Can you work these out from the model? Positions are in its coordinate system, mm. A direction names the side the tool comes from. Round coordinates to 2 decimals unless told otherwise and drop trailing zeros. Order: outer loops, then holes, each group sorted by start corner. A loop starts at its lowest first (then second) coordinate and runs counter-clockwise, first axis right, second up. Notation, with made-up numbers: M -23,69 L -7,69 A17 ccw -7,94 Z; hole C -38.75,-34 d7. An arc over 180 degrees is marked long. Answer as a JSON object with one key per item and string values. Group by question number.
```python
from build123d import *

# Parameters (mm, degrees)
SKETCH2_R           = 7.5
BOSS_EXTRUDE1_DEPTH = 8
BOSS_EXTRUDE3_DEPTH = 8
SKETCH3_4_R         = 25
SKETCH3_4_R_2       = 15
BOSS_EXTRUDE4_DEPTH = 58
SKETCH17_W          = 8
SKETCH17_H          = 39.501765498
BOSS_EXTRUDE6_DEPTH = 78
CUT_EXTRUDE1_DEPTH  = 78


with BuildPart() as part:
    # Sketch2 → Boss-Extrude1 (new body)
    with BuildSketch(Plane(origin=(0, 0, 0), x_dir=(1, 0, 0), z_dir=(0, 1, 0))):
        with BuildLine():
            Line((-4.545115865, -26.622255639), (58.454884135, -26.622255639))
            ThreePointArc((58.454884135, -26.622255639), (69.061485853, -22.228857357), (73.454884135, -11.622255639))
            Line((73.454884135, -11.622255639), (73.454884135, 48.377744361))
            ThreePointArc((73.454884135, 48.377744361), (69.061485853, 58.984346079), (58.454884135, 63.377744361))
            Line((58.454884135, 63.377744361), (-4.545115865, 63.377744361))
            Line((-4.545115865, 63.377744361), (-4.545115865, -26.622255639))
        make_face()
        with Locations((58.454884135, -11.622255639)):
            Circle(SKETCH2_R, mode=Mode.SUBTRACT)
        with Locations((58.454884135, 48.377744361)):
            Circle(SKETCH2_R, mode=Mode.SUBTRACT)
    extrude(amount=BOSS_EXTRUDE1_DEPTH)

    # Sketch3 → Boss-Extrude3 (add)
    with BuildSketch(Plane.ZY.offset(4.545115865)):
        with BuildLine():
            Line((-18.377744361, 42), (-18.377744361, 8))
            Line((-18.377744361, 8), (26.622255639, 8))
            Line((26.622255639, 8), (6.622255639, 67))
            ThreePointArc((6.622255639, 67), (-0.700074831, 49.32233047), (-18.377744361, 42))
        make_face()
        with BuildLine():
            Line((-63.377744361, 8), (-18.377744361, 8))
            Line((-18.377744361, 8), (-18.377744361, 42))
            ThreePointArc((-18.377744361, 42), (-36.055413891, 49.32233047), (-43.377744361, 67))
            Line((-43.377744361, 67), (-63.377744361, 8))
        make_face()
    extrude(amount=-BOSS_EXTRUDE3_DEPTH)

    # Sketch3_4 → Boss-Extrude4 (add)
    with BuildSketch(Plane.ZY.offset(4.545115865)):
        with Locations((-18.377744361, 67)):
            Circle(SKETCH3_4_R)
        with Locations((-18.377744361, 67)):
            Circle(SKETCH3_4_R_2, mode=Mode.SUBTRACT)
    extrude(amount=-BOSS_EXTRUDE4_DEPTH)

    # Sketch17 → Boss-Extrude6 (add)
    with BuildSketch(Plane.ZY.offset(4.545115865)):
        with Locations((-18.377744361, 27.750882749)):
            Rectangle(SKETCH17_W, SKETCH17_H)
    extrude(amount=-BOSS_EXTRUDE6_DEPTH)

    # Sketch18 → Cut-Extrude1 (cut)
    with BuildSketch(Plane(origin=(0, 0, -22.377744361), x_dir=(-1, 0, 0), z_dir=(0, 0, -1))):
        Polygon((-73.454884135, 8), (-53.454884135, 42.322074641), (-53.454884135, 47.501765498), (-73.454884135, 47.501765498), align=None)
    extrude(amount=-CUT_EXTRUDE1_DEPTH, mode=Mode.SUBTRACT)


solid = part.part
```
1) Which directions (+Z, -Z, +X, -X, +Y, -Y) give clear straight access to the entire face, cutting with the end or side of a thin tool? Please do faces 4 (the face through (24.05, 91.98, -17.33)), 5 (the face through (3.455, 31, -39)), 6 (the face through (30, 25, -14.378)).
2) For pin 1 (6 mm diameter, centred on x = 9, y = 45, fed in from +Z); pin 2 (20.5 mm diameter, centred on y = 33.5, z = -40, fed in from +X); pin 3 (18 mm diameter, centred on y = 67, z = -18.38, fed in from -X); pin 4 (17 mm diameter, centred on x = 43.5, y = 20, fed in from -Z), each with a flat end and sliding along its axis, tell me the tip position at first contact or that it passes through.
3) If we section it at B-B on z = -11.5: Write out the boundary of the cut face in (x, y), plus the area to 3 significant figures.
4) We'd pull the mould along Y, two halves only. Please class faces 1 (the face through (-0.6, 37.91, -53.24)), 2 (the face through (34, 0, -19)), 3 (the face through (24.049, 52.357, -21.629)): +Y half, -Y half, draft (parallel to the pull), parting line (faces both ways), or undercut.
5) If we section it at C-C on y = 75: Write out the boundary of the cut face in (x, z), plus the area to 3 significant figures.
6) If we section it at A-A on x = 6.5: Write out the boundary of the cut face in (y, z).
7) I need wall thicknesses on line 1 along Y through (x, z) = (4, -24); line 2 along Y through (x, z) = (24.5, -28); line 3 along X through (y, z) = (33, -27.5). Which ranges of each line are inside material? Lowest first, please.
8) If we section it at D-D on x = 55: Write out the boundary of the cut face in (y, z), plus the area to 3 significant figures.
Findings:
{
 "1": {"face 4": "+X", "face 5": "-Z, +X", "face 6": "+Z, +X"},
 "2": {"pin 1": "stops at z = -2.13", "pin 2": "stops at x = 3.45", "pin 3": "passes through", "pin 4": "stops at z = -22.38"},
 "3": {"outline": "M -4.55,0 L 73.45,0 L 73.45,8 L 3.45,8 L 3.45,42.96 L 53.45,42.96 L 53.45,53.67 L -4.55,53.67 Z; M -4.55,80.33 L 53.45,80.33 L 53.45,91.04 L -4.55,91.04 Z", "area": "2,150 mm^2"},
 "4": {"face 1": "+Y half", "face 2": "-Y half", "face 3": "undercut"},
 "5": {"outline": "M -4.55,-42.06 L 53.45,-42.06 L 53.45,-31.07 L -4.55,-31.07 Z; M -4.55,-5.69 L 53.45,-5.69 L 53.45,5.31 L -4.55,5.31 Z", "area": "1,280 mm^2"},
 "6": {"outline": "M 0,-63.38 L 8,-63.38 L 8,-22.38 L 42.32,-22.38 A25 ccw long 42.32,-14.38 L 8,-14.38 L 8,26.62 L 0,26.62 Z; hole C 67,-18.38 d30"},
 "7": {"line 1": "y = 0 to 8, 42.64 to 53.09, 80.91 to 91.36", "line 2": "y = 0 to 8, 43.93 to 55.49, 78.51 to 90.07", "line 3": "x = -4.55 to 3.45"},
 "8": {"outline": "M 0,-63.38 L 8,-63.38 L 8,-55.03 L 0,-55.03 Z; M 0,-41.72 L 8,-41.72 L 8,-22.38 L 39.67,-22.38 L 39.67,-14.38 L 8,-14.38 L 8,4.97 L 0,4.97 Z; M 0,18.28 L 8,18.28 L 8,26.62 L 0,26.62 Z", "area": "760 mm^2"}
}
